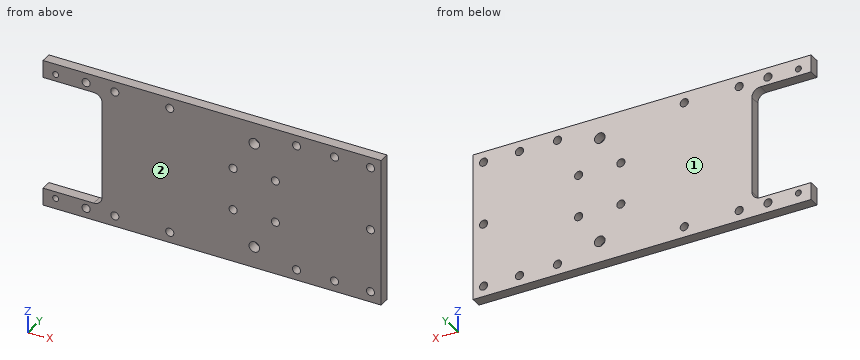
from build123d import *

# Parameters (mm, degrees)
SKETCH1_W           = 101.6
SKETCH1_H           = 44.45
BOSS_EXTRUDE1_DEPTH = 3.175
SKETCH2_R           = 0.889
SKETCH2_R_2         = 1.2192
CUT_EXTRUDE1_DEPTH  = 56.539816798
SKETCH3_R           = 1.2192
SKETCH3_R_2         = 1.5875
CUT_EXTRUDE2_DEPTH  = 56.539816798
SKETCH4_W           = 17.78
SKETCH4_H           = 34.036
CUT_EXTRUDE3_DEPTH  = 56.539816798
FILLET2_R           = 2.54


with BuildPart() as part:
    # Sketch1 → Boss-Extrude1 (new body)
    with BuildSketch(Plane(origin=(0, 0, 0), x_dir=(1, 0, 0), z_dir=(0, 1, 0))):
        Rectangle(SKETCH1_W, SKETCH1_H)
    extrude(amount=BOSS_EXTRUDE1_DEPTH)

    # Sketch2 → Cut-Extrude1 (cut, through all)
    with BuildSketch(Plane(origin=(0, 3.175, 0), x_dir=(1, 0, 0), z_dir=(0, 1, 0))):
        with Locations(Location((-46.99, 19.05, 0), (0, 0, 270))):
            Circle(SKETCH2_R)
        with Locations(Location((-29.21, 19.05, 0), (0, 0, 270))):
            Circle(SKETCH2_R_2)
        with Locations(Location((-12.7, 19.05, 0), (0, 0, 270))):
            Circle(SKETCH2_R_2)
        with Locations(Location((25.4, 19.05, 0), (0, 0, 270))):
            Circle(SKETCH2_R_2)
        with Locations(Location((36.83, 19.05, 0), (0, 0, 270))):
            Circle(SKETCH2_R_2)
        with Locations(Location((47.625, 19.05, 0), (0, 0, 270))):
            Circle(SKETCH2_R_2)
        with Locations(Location((47.625, 0, 0), (0, 0, 270))):
            Circle(SKETCH2_R_2)
        with Locations(Location((47.625, -19.05, 0), (0, 0, 270))):
            Circle(SKETCH2_R_2)
        with Locations(Location((36.83, -19.05, 0), (0, 0, 270))):
            Circle(SKETCH2_R_2)
        with Locations(Location((25.4, -19.05, 0), (0, 0, 270))):
            Circle(SKETCH2_R_2)
        with Locations(Location((-12.7, -19.05, 0), (0, 0, 270))):
            Circle(SKETCH2_R_2)
        with Locations(Location((-29.21, -19.05, 0), (0, 0, 270))):
            Circle(SKETCH2_R_2)
        with Locations(Location((-46.99, -19.05, 0), (0, 0, 270))):
            Circle(SKETCH2_R)
        with Locations(Location((19.05, -6.35, 0), (0, 0, 270))):
            Circle(SKETCH2_R_2)
        with Locations(Location((19.05, 6.35, 0), (0, 0, 270))):
            Circle(SKETCH2_R_2)
        with Locations(Location((6.35, 6.35, 0), (0, 0, 270))):
            Circle(SKETCH2_R_2)
        with Locations(Location((6.35, -6.35, 0), (0, 0, 270))):
            Circle(SKETCH2_R_2)
    extrude(amount=-CUT_EXTRUDE1_DEPTH, mode=Mode.SUBTRACT)

    # Sketch3 → Cut-Extrude2 (cut, through all)
    with BuildSketch(Plane(origin=(0, 3.175, 0), x_dir=(1, 0, 0), z_dir=(0, 1, 0))):
        with Locations(Location((-37.846, 19.3294, 0), (0, 0, 270))):
            Circle(SKETCH3_R)
        with Locations(Location((12.7, 15.875, 0), (0, 0, 270))):
            Circle(SKETCH3_R_2)
    cut_extrude2 = extrude(amount=-CUT_EXTRUDE2_DEPTH, mode=Mode.SUBTRACT)

    # Mirror1: Cut-Extrude2 across plane
    add(cut_extrude2.mirror(Plane.XY), mode=Mode.SUBTRACT)

    # Sketch4 → Cut-Extrude3 (cut, through all)
    with BuildSketch(Plane(origin=(0, 3.175, 0), x_dir=(1, 0, 0), z_dir=(0, 1, 0))):
        with Locations((-41.91, 0)):
            Rectangle(SKETCH4_W, SKETCH4_H)
    extrude(amount=-CUT_EXTRUDE3_DEPTH, mode=Mode.SUBTRACT)

    # Fillet2
    fillet2_edges = [part.edges().sort_by_distance(p)[0] for p in [
        (-33.02, 1.5875, -17.018),
        (-33.02, 1.5875, 17.018),
    ]]
    fillet(fillet2_edges, radius=FILLET2_R)


solid = part.part
Source: CAD feature listing. Evaluate the final solid. Frame: model axes, mm. Face numbers are marked on the shaded views. Coordinates: 2 decimals unless noted, no trailing zeros. Order: outer loops, then holes, each group sorted by start corner. A loop starts at its lowest first (then second) coordinate and runs counter-clockwise, first axis right, second up. Notation, with made-up numbers: M 8,64 L 29,64 A34 cw 29,99 Z; hole C -9,28 d3. An arc over 180 degrees is marked long. Write each question's results on one line, items separated by ' | '. Start each with the question number.
Item 1: Cut plane C-C (x = -46.99). Return loops of the section in (y, z) (3 decimals), and give its area (3 significant figures).
Item 2: Cut plane A-A (z = 6.35). Return loops of the section in (x, y) (3 decimals), and give its area (3 significant figures).
Item 3: Draft query along Y for the marked faces 1 and 2. Return one class per face: pulls with the +Y half, pulls with the -Y half, needs draft (parallel to the pull), parting line crosses it, or undercut.
Item 4: Line query: probe 1 along Z at (x, y) = (12.5, 2.65) (3 decimals); probe 2 along X at (y, z) = (1.3, 6.35); probe 3 along Z at (x, y) = (19, 0.15) (3 decimals). Output: solid intervals per line, ascending.
Item 5: First-contact query: pin 1 Ø1.5 at (x, z) = (19.05, -6.35) entering from +Y; pin 2 Ø1.6 at (y, z) = (1, 5) entering from -X. Flat tips, straight axial feed; report the tip coordinate or a pass-through.
Item 6: Cut plane D-D (z = 0). Return loops of the section in (x, y) (3 decimals).
Item 7: Cut plane B-B (x = -29.21). Return loops of the section in (y, z) (3 decimals).
Checked values:
1) outline: M 0,-22.225 L 3.175,-22.225 L 3.175,-19.939 L 0,-19.939 Z; M 0,-18.161 L 3.175,-18.161 L 3.175,-17.018 L 0,-17.018 Z; M 0,17.018 L 3.175,17.018 L 3.175,18.161 L 0,18.161 Z; M 0,19.939 L 3.175,19.939 L 3.175,22.225 L 0,22.225 Z | area: 21.8 mm2
2) outline: M -33.02,0 L 5.131,0 L 5.131,3.175 L -33.02,3.175 Z; M 7.569,0 L 17.831,0 L 17.831,3.175 L 7.569,3.175 Z; M 20.269,0 L 50.8,0 L 50.8,3.175 L 20.269,3.175 Z | area: 251 mm2
3) face 1: pulls with the +Y half | face 2: pulls with the -Y half
4) probe 1: z = -22.225 to -17.45, -14.3 to 14.3, 17.45 to 22.225 | probe 2: x = -33.02 to 5.13, 7.57 to 17.83, 20.27 to 50.8 | probe 3: z = -22.225 to -7.568, -5.132 to 5.132, 7.568 to 22.225
5) pin 1: passes through | pin 2: stops at x = -33.02
6) outline: M -33.02,0 L 46.406,0 L 46.406,3.175 L -33.02,3.175 Z; M 48.844,0 L 50.8,0 L 50.8,3.175 L 48.844,3.175 Z
7) outline: M 0,-22.225 L 3.175,-22.225 L 3.175,-20.269 L 0,-20.269 Z; M 0,-17.831 L 3.175,-17.831 L 3.175,17.831 L 0,17.831 Z; M 0,20.269 L 3.175,20.269 L 3.175,22.225 L 0,22.225 Z
